from build123d import *

# Parameters (mm, degrees)
SKETCH1_R           = 18.75
BOSS_EXTRUDE1_DEPTH = 15
BOSS_EXTRUDE2_START = -15
BOSS_EXTRUDE2_DEPTH = 15
CIRPATTERN1_COUNT   = 16
SKETCH3_R           = 6
CUT_EXTRUDE1_DEPTH  = 41.039043445
SKETCH4_R           = 12.5
CUT_EXTRUDE2_DEPTH  = 7.5


with BuildPart() as part:
    # Sketch1 → Boss-Extrude1 (new body)
    with BuildSketch(Plane(origin=(0, 0, 0), x_dir=(1, 0, 0), z_dir=(0, 1, 0))):
        with Locations(Location((0, 0, 0), (0, 0, 270))):
            Circle(SKETCH1_R)
    extrude(amount=BOSS_EXTRUDE1_DEPTH)

    # Sketch2 → Boss-Extrude2 (add)
    with BuildSketch(Plane(origin=(0, 15, 0), x_dir=(1, 0, 0), z_dir=(0, 1, 0)).offset(BOSS_EXTRUDE2_START)):
        with BuildLine():
            Line((-1.25, 26.25), (1.25, 26.25))
            Line((1.25, 26.25), (2.203742352, 18.620043492))
            ThreePointArc((2.203742352, 18.620043492), (0, 18.75), (-2.203742352, 18.620043492))
            Line((-2.203742352, 18.620043492), (-1.25, 26.25))
        make_face()
    boss_extrude2 = extrude(amount=BOSS_EXTRUDE2_DEPTH)

    # CirPattern1: Boss-Extrude2 ×16 about axis
    cirpattern1_axis = Axis((0, 0, 0), (0, 1, 0))
    for i in range(1, CIRPATTERN1_COUNT):
        add(boss_extrude2.rotate(cirpattern1_axis, i * 360 / CIRPATTERN1_COUNT))

    # Sketch3 → Cut-Extrude1 (cut, through all)
    with BuildSketch(Plane(origin=(0, 15, 0), x_dir=(1, 0, 0), z_dir=(0, 1, 0))):
        with Locations(Location((0, 0, 0), (0, 0, 270))):
            Circle(SKETCH3_R)
    extrude(amount=-CUT_EXTRUDE1_DEPTH, mode=Mode.SUBTRACT)

    # Sketch4 → Cut-Extrude2 (cut)
    with BuildSketch(Plane(origin=(0, 0, 0), x_dir=(-1, 0, 0), z_dir=(0, -1, 0))):
        with Locations(Location((0, 0, 0), (0, 0, 90))):
            Circle(SKETCH4_R)
    extrude(amount=-CUT_EXTRUDE2_DEPTH, mode=Mode.SUBTRACT)


solid = part.part
The model under review builds one solid part; all positions refer to its coordinate system, in mm. A direction names the side the tool comes from. Give positions to 0.01 mm unless a question says otherwise; leave off trailing zeros. Loops run counter-clockwise (first coordinate to the right, second up) from the corner with the lowest first, then second, coordinate; pieces in that order, holes last. Notation, with made-up numbers: (75, -25.75) -> (110, -25.75) arc R29 ccw to (110, 0.25) -> close; hole circle Ø7 at (36, 26.25). An arc over 180 degrees is marked (long way). Answer as a JSON object with one key per item and string values. Group by question number.
Q1. Take a section at B-B (z = 0). Write out the cut boundary in (x, y), plus the area to 3 significant figures.
Q2. Take a section at A-A (x = 0). Write out the cut boundary in (y, z), plus the area to 3 significant figures.
Q3. Draft analysis for pull direction Z (two halves, no side actions). For faces 5 (the flat face through (26.25, 7, 0)), 6 (the cylindrical face through (-3.6, 7.4, -18.4)), 7 (the flat face through (-22.49, 7.4, -1.72)), state which applies: pulls with the +Z half, pulls with the -Z half, needs draft (parallel to the pull), parting line crosses it, or undercut.
Q4. Insertion check: pin 1 (1.5 mm diameter, centred on y = 3, z = -20.5, fed in from +X); pin 2 (20 mm diameter, centred on x = 0, z = 0, fed in from -Y); pin 3 (7.5 mm diameter, centred on x = -0.5, z = -1.5, fed in from -Y); pin 4 (1 mm diameter, centred on y = 12, z = 16, fed in from +X). Each pin has a flat end and moves straight along its axis. Give the tip position at first contact, or say it passes through.
Q5. Wall thickness on line 1 along X through (y, z) = (13.25, 0); line 2 along Z through (x, y) = (-15, 6); line 3 along X through (y, z) = (5, 17): over which ranges is each line inside the solid? List them lowest first.
Q6. Tool access review of faces 1 (the cylindrical face through (3.755, 3.698, -11.923)), 2 (the cylindrical face through (-18.4, 7.4, 3.6)), 3 (the cylindrical face through (10.4, 7.4, -15.6)), 4 (the flat face through (17.12, 7.4, -14.69)): name each direction out of +Z, -Z, +X, -X, +Y, -Y from which nothing blocks a thin tool from reaching the whole face with its end or side.
Q7. Take a section at C-C (z = -17). Write out the cut boundary in (x, y).
Answer below:
{
 "1": {"outline": "(-26.25, 0) -> (-12.5, 0) -> (-12.5, 7.5) -> (-6, 7.5) -> (-6, 15) -> (-26.25, 15) -> close; (6, 7.5) -> (12.5, 7.5) -> (12.5, 0) -> (26.25, 0) -> (26.25, 15) -> (6, 15) -> close", "area": "510 mm2"},
 "2": {"outline": "(0, -26.25) -> (15, -26.25) -> (15, -6) -> (7.5, -6) -> (7.5, -12.5) -> (0, -12.5) -> close; (0, 12.5) -> (7.5, 12.5) -> (7.5, 6) -> (15, 6) -> (15, 26.25) -> (0, 26.25) -> close", "area": "510 mm2"},
 "3": {"face 5": "needs draft", "face 6": "pulls with the -Z half", "face 7": "undercut"},
 "4": {"pin 1": "stops at x = 10.51", "pin 2": "stops at y = 7.5", "pin 3": "passes through", "pin 4": "stops at x = 18.53"},
 "5": {"line 1": "x = -26.25 to -6, 6 to 26.25", "line 2": "z = -17.36 to -11.96, -11.25 to 11.25, 11.96 to 17.36", "line 3": "x = -18.92 to -14.53, -9.34 to 9.34, 14.53 to 18.92"},
 "6": {"face 1": "-Y", "face 2": "-X, +Y, -Y", "face 3": "+Y, -Y", "face 4": "+X, +Y, -Y"},
 "7": {"outline": "(-18.92, 0) -> (-14.53, 0) -> (-14.53, 15) -> (-18.92, 15) -> close; (-9.34, 0) -> (9.34, 0) -> (9.34, 15) -> (-9.34, 15) -> close; (14.53, 0) -> (18.92, 0) -> (18.92, 15) -> (14.53, 15) -> close"}
}
